Autodesk Inventor part; units mm, degrees
ref_plane "YZ Plane" through (0, 0, 0) normal (1, 0, 0) x (0, 1, 0)
ref_plane "XZ Plane" through (0, 0, 0) normal (0, 1, 0) x (-1, 0, 0)
ref_plane "XY Plane" through (0, 0, 0) normal (0, 0, 1) x (1, 0, 0)
sketch "Эскиз1" plane through (0, 0, 0) normal (0, 1, 0) x (-1, 0, 0)
  circle A0 centre (0, 0) radius 3.5
  circle A1 centre (0, -8.5) radius 1.5
  circle A2 centre (6.0104, -6.0104) radius 1.5
  circle A3 centre (8.5, 0) radius 1.5
  circle A4 centre (6.0104, 6.0104) radius 1.5
  circle A5 centre (0, 8.5) radius 1.5
  circle A6 centre (-6.0104, 6.0104) radius 1.5
  circle A7 centre (-8.5, 0) radius 1.5
  circle A8 centre (-6.0104, -6.0104) radius 1.5
  line L0 (17.5, 17.5) -> (-17.5, 17.5)
  line L1 (-17.5, 17.5) -> (-17.5, -17.5)
  line L2 (-17.5, -17.5) -> (17.5, -17.5)
  line L3 (17.5, -17.5) -> (17.5, 17.5)
  dimension "d0" = 7
  dimension "d1" = 3
  dimension "d2" = 8.5
  dimension "d5" = 360
  dimension "d7" = 35
  dimension "d8" = 17.5
  dimension "d9" = 35
  dimension "d10" = 17.5
extrude "Выдавливание1" add sketch "Эскиз1" along normal blind 1
sketch "Эскиз2" plane through (0, 1, 0) normal (0, 1, 0) x (1, 0, 0)
  circle A0 centre (0, 0) radius 3.5
  circle A1 centre (6.0104, 6.0104) radius 1.5
  circle A2 centre (8.5, 0) radius 1.5
  circle A3 centre (6.0104, -6.0104) radius 1.5
  circle A4 centre (0, -8.5) radius 1.5
  circle A5 centre (-6.0104, -6.0104) radius 1.5
  circle A6 centre (-8.5, 0) radius 1.5
  circle A7 centre (-6.0104, 6.0104) radius 1.5
  circle A8 centre (0, 8.5) radius 1.5
  line L0 (-17.5, -17.5) -> (17.5, -17.5)
  line L1 (17.5, -17.5) -> (17.5, 17.5)
  line L2 (17.5, 17.5) -> (-17.5, 17.5)
  line L3 (-17.5, 17.5) -> (-17.5, -17.5)
  line L4 (-16.5, -16.5) -> (16.5, -16.5)
  line L5 (16.5, -16.5) -> (16.5, 16.5)
  line L6 (16.5, 16.5) -> (-16.5, 16.5)
  line L7 (-16.5, 16.5) -> (-16.5, -16.5)
  dimension "d13" = 1
  dimension "d14" = 1
  dimension "d15" = 1
  dimension "d16" = 1
extrude "Выдавливание2" add sketch "Эскиз2" along normal blind 12 contours L3 L2 L1 L0
sketch "Эскиз3" plane through (17.5, 0, 17.5) normal (1, 0, 0) x (0, 0, -1)
  circle A0 centre (17.5, 6.5) radius 2
  line L0 (0, 0) -> (0, 13)
  line L1 (35, 0) -> (35, 13)
  line L2 (0, 0) -> (35, 0)
  line L3 (0, 13) -> (35, 13)
  circle A1 centre (27.5, 6.5) radius 2
  circle A2 centre (7.5, 6.5) radius 2
  point P0 (17.5, 0)
  dimension "d19" = 4
  dimension "d20" = 35
  dimension "d21" = 17.5
  dimension "d22" = 13
  dimension "d23" = 6.5
  dimension "d24" = 4
  dimension "d25" = 10
  dimension "d26" = 4
  dimension "d27" = 10
extrude "Выдавливание3" cut sketch "Эскиз3" against normal blind 40 contours A0 | A1 | A2
sketch "Эскиз4" plane through (-17.5, 0, 17.5) normal (0, 0, 1) x (1, 0, 0)
  circle A0 centre (17.5, 6.5) radius 2
  line L0 (35, 0) -> (35, 13)
  line L1 (0, 0) -> (0, 13)
  line L2 (0, 0) -> (35, 0)
  line L3 (0, 13) -> (35, 13)
  circle A1 centre (27.5, 6.5) radius 2
  circle A2 centre (7.5, 6.5) radius 2
  point P0 (17.5, 0)
  dimension "d30" = 4
  dimension "d31" = 35
  dimension "d32" = 13
  dimension "d33" = 6.5
  dimension "d34" = 17.5
  dimension "d35" = 4
  dimension "d36" = 10
  dimension "d39" = 360
extrude "Выдавливание4" cut sketch "Эскиз4" against normal blind 40 contours A0 | A1 | A2
equation "\"d9\" = d7"
equation "\"d10\" = 0.5 * d9"
equation "\"d14\" = d13"
equation "\"d15\" = d13"
equation "\"d16\" = d13"
equation "\"d21\" = 0.5 * d20"
equation "\"d23\" = 0.5 * d22"
equation "\"d33\" = 0.5 * d32"
equation "\"d34\" = 0.5 * d31"
properties part number "01_Крепление_мотора" material "Сталь"
Source: CAD feature listing. Evaluate the final solid. Frame: model axes, mm. A direction names the side the tool comes from. Round coordinates to 2 decimals unless told otherwise and drop trailing zeros. Loops run counter-clockwise (first coordinate to the right, second up) from the corner with the lowest first, then second, coordinate; pieces in that order, holes last. Notation, with made-up numbers: M -9.5,18.5 L 8.5,18.5 A17 ccw 8.5,32.5 Z; hole C 26.25,-31.5 d9. An arc over 180 degrees is marked long. Use a Markdown table: item, result. Add a question column.
1. Contact query for a flat-ended pin moving along its axis: pin 1 (3.5 mm diameter, centred on x = -6.01, z = -6.01, fed in from +Y). Output: stop coordinate, or through.
2. Cut plane A-A, the plane x = 0. Output: boundary loops of the cut face in (y, z).
3. Pull-direction query (Z, two-part tool) for faces 3 (the flat face through (-17.5, 4, 0)), 4 (the cylindrical face through (5.32, 0.49, 7.34)), 5 (the flat face through (0, 4, 17.5)); classes: +Z half, -Z half, draft (parallel to the pull), parting line (faces both ways), or undercut.
4. Set-up query: faces 1 (the cylindrical face through (-4.82, 0.49, 6.92)), 2 (the flat face through (0, 10, -16.5)). Return all of +Z, -Z, +X, -X, +Y, -Y with unobstructed straight access to the full face (end or side cutting, diameter ignored); none if empty.
5. Cut plane D-D, the plane z = 8.5. Output: boundary loops of the cut face in (x, y), and give its area (3 significant figures).
6. Cut plane C-C, the plane z = 0. Output: boundary loops of the cut face in (x, y), and give its area (3 significant figures).
7. Cut plane B-B, the plane y = 2.5. Output: boundary loops of the cut face in (x, z), and give its area (3 significant figures).
8. Ray query, line 1 along Z through (x, y) = (0, 0.75); line 2 along X through (y, z) = (10.25, -11.5). Return the intervals inside material, ascending. Write a range as [from, to].
Solution:
| question | item | result |
|---|---|---|
| 1 | pin 1 | stops at y = 1 |
| 2 | outline | M 0,-17.5 L 4.5,-17.5 L 4.5,-16.5 L 1,-16.5 L 1,-10 L 0,-10 Z; M 0,-7 L 1,-7 L 1,-3.5 L 0,-3.5 Z; M 0,3.5 L 1,3.5 L 1,7 L 0,7 Z; M 0,10 L 1,10 L 1,16.5 L 4.5,16.5 L 4.5,17.5 L 0,17.5 Z; M 8.5,-17.5 L 13,-17.5 L 13,-16.5 L 8.5,-16.5 Z; M 8.5,16.5 L 13,16.5 L 13,17.5 L 8.5,17.5 Z |
| 3 | face 3 | draft |
| 3 | face 4 | undercut |
| 3 | face 5 | +Z half |
| 4 | face 1 | +Y, -Y |
| 4 | face 2 | +Y |
| 5 | outline | M -17.5,0 L -1.5,0 L -1.5,1 L -16.5,1 L -16.5,5.18 L -17.5,5.18 Z; M -17.5,7.82 L -16.5,7.82 L -16.5,13 L -17.5,13 Z; M 1.5,0 L 17.5,0 L 17.5,5.18 L 16.5,5.18 L 16.5,1 L 1.5,1 Z; M 16.5,7.82 L 17.5,7.82 L 17.5,13 L 16.5,13 Z |
| 5 | area | 50.7 mm2 |
| 6 | outline | M -17.5,0 L -10,0 L -10,1 L -16.5,1 L -16.5,4.5 L -17.5,4.5 Z; M -17.5,8.5 L -16.5,8.5 L -16.5,13 L -17.5,13 Z; M -7,0 L -3.5,0 L -3.5,1 L -7,1 Z; M 3.5,0 L 7,0 L 7,1 L 3.5,1 Z; M 10,0 L 17.5,0 L 17.5,4.5 L 16.5,4.5 L 16.5,1 L 10,1 Z; M 16.5,8.5 L 17.5,8.5 L 17.5,13 L 16.5,13 Z |
| 6 | area | 38.0 mm2 |
| 7 | outline | M -17.5,-17.5 L 17.5,-17.5 L 17.5,17.5 L -17.5,17.5 Z; hole M -16.5,-16.5 L 16.5,-16.5 L 16.5,16.5 L -16.5,16.5 Z |
| 7 | area | 136 mm2 |
| 8 | line 1 | z = [-17.5, -10], [-7, -3.5], [3.5, 7], [10, 17.5] |
| 8 | line 2 | x = [-17.5, -16.5], [16.5, 17.5] |
